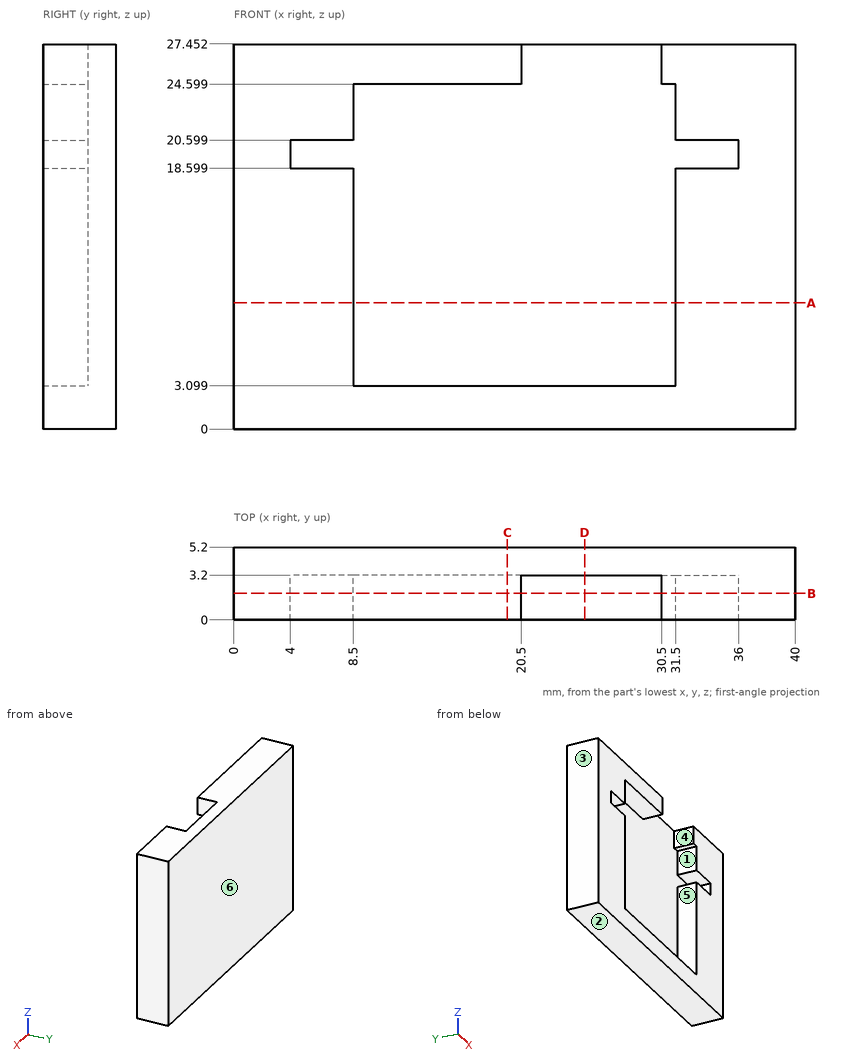
Source: three-view drawing plus pictorial views. Frame: mm from the lowest corner of the part. A direction names the side the tool comes from. Coordinates: 2 decimals unless noted, no trailing zeros. Write each loop counter-clockwise with the first axis right and the second up, starting at its lowest first coordinate (ties: lowest second). Pieces come first, ordered by that corner, then holes. Notation, with made-up numbers: (-36, 32.5) -> (12, 32.5) arc R9 ccw to (12, 39.5) -> close; hole circle Ø7 at (-20, 22.25). An arc over 180 degrees is marked (long way). Write each question's results on one line, items separated by ' | '.
Item 1: Section query D-D on x = 25. Return loops of the section in (y, z).
Conclusion:
outline: (0, 0) -> (5.2, 0) -> (5.2, 27.45) -> (3.2, 27.45) -> (3.2, 3.1) -> (0, 3.1) -> close
Item 2: Mould query, pull axis Z, two halves, no side actions, for the marked faces 1, 2 and 3. Classes: +Z half, -Z half, draft (parallel to the pull), parting line (faces both ways), or undercut.
Conclusion:
face 1: undercut | face 2: -Z half | face 3: draft
Item 3: Section query B-B on y = 1.9. Return loops of the section in (x, z), plus the area to 3 significant figures.
Conclusion:
outline: (0, 0) -> (40, 0) -> (40, 27.45) -> (30.5, 27.45) -> (30.5, 24.6) -> (31.5, 24.6) -> (31.5, 20.6) -> (36, 20.6) -> (36, 18.6) -> (31.5, 18.6) -> (31.5, 3.1) -> (8.5, 3.1) -> (8.5, 18.6) -> (4, 18.6) -> (4, 20.6) -> (8.5, 20.6) -> (8.5, 24.6) -> (20.5, 24.6) -> (20.5, 27.45) -> (0, 27.45) -> close | area: 557 mm^2
Item 4: Set-up query: the marked faces 4, 5 and 6. Return all of +Z, -Z, +X, -X, +Y, -Y with unobstructed straight access to the full face (end or side cutting, diameter ignored); none if empty.
Conclusion:
face 4: +Z, -Y | face 5: -Y | face 6: +Z, -Z, +X, -X, +Y
Item 5: Pin query (flat end, axial travel): pin 1 Ø1.4 at (y, z) = (2, 26.5) entering from -X; pin 2 Ø12 at (x, z) = (18.5, 15) entering from -Y. Return the tip coordinate at first contact, or that it passes through.
Conclusion:
pin 1: stops at x = 0 | pin 2: stops at y = 3.2
Item 6: Section query A-A on z = 9. Return loops of the section in (x, y).
Conclusion:
outline: (0, 0) -> (8.5, 0) -> (8.5, 3.2) -> (31.5, 3.2) -> (31.5, 0) -> (40, 0) -> (40, 5.2) -> (0, 5.2) -> close
Item 7: Material intervals for probe 1 along X at (y, z) = (1.6, 18); probe 2 along X at (y, z) = (1.85, 26.25); probe 3 along Z at (x, y) = (13.5, 1.45), sorted ascending.
Conclusion:
probe 1: x = 0 to 8.5, 31.5 to 40 | probe 2: x = 0 to 20.5, 30.5 to 40 | probe 3: z = 0 to 3.1, 24.6 to 27.45
Item 8: Section query C-C on x = 19.5. Return loops of the section in (y, z).
Conclusion:
outline: (0, 0) -> (5.2, 0) -> (5.2, 27.45) -> (0, 27.45) -> (0, 24.6) -> (3.2, 24.6) -> (3.2, 3.1) -> (0, 3.1) -> close
